from build123d import *

# Parameters (mm, degrees)
F0_R     = 68.9341581071
F1_DEPTH = 6.35
F2_R     = 25.775239711
F3_DEPTH = 3.81
F5_R     = 16.9134232358
F6_DEPTH = 3.81


# Not quite as in the source:
# - a feature names something its author has since deleted; it is built from what else it names


with BuildPart() as f1:
    # F0 (on Top) → F1 (new body)
    with BuildSketch(Plane.XY):
        Circle(F0_R)
    extrude(amount=F1_DEPTH)

    # F2 (on face) → F3 (cut)
    with BuildSketch(Plane.XY.offset(6.35)):
        Circle(F2_R)
    extrude(amount=-F3_DEPTH, mode=Mode.SUBTRACT)

    # F5 (on face) → F6 (cut)
    with BuildSketch(Plane.XY.offset(6.35)):
        with Locations((-42.6894489161, -25.2584252012)):
            Circle(F5_R)
        with Locations((-37.2139550745, 32.7947959304)):
            Circle(F5_R)
        with Locations((19.6899598242, 45.5267237403)):
            Circle(F5_R)
        with Locations((49.383019483, -4.6577332624)):
            Circle(F5_R)
        with Locations((10.8304246834, -48.405361207)):
            Circle(F5_R)
    extrude(amount=-F6_DEPTH, mode=Mode.SUBTRACT)


solid = f1.part
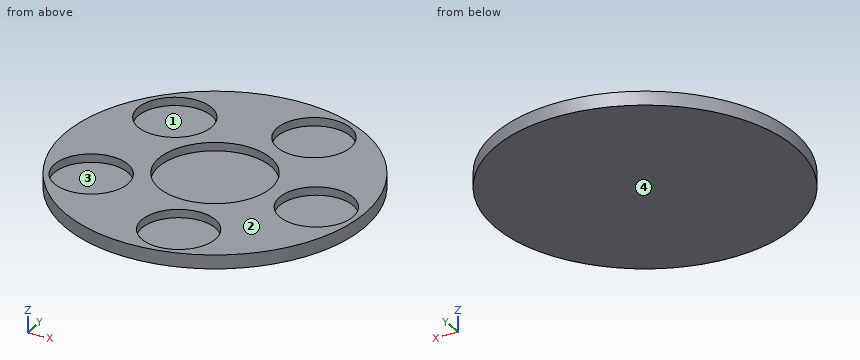
CAD build for the part. Positions are in the model's coordinates, mm. Face numbers are marked on the shaded views. A direction names the side the tool comes from. Give positions to 0.01 mm unless a question says otherwise; leave off trailing zeros. Order: outer loops, then holes, each group sorted by start corner. A loop starts at its lowest first (then second) coordinate and runs counter-clockwise, first axis right, second up. Notation, with made-up numbers: (-22.75, 77.5) - (5.25, 77.5) arc R10 cw to (5.25, 82.5) - close; hole circle Ø4 at (16.25, -36.5). An arc over 180 degrees is marked (long way). Answer in a Markdown table with one row per item.
1. Saw through at A-A, the plane z = 4.75. Give the cut face in (x, y), plus the area to 3 significant figures.
Data:
| item | result |
|---|---|
| outline | circle Ø137.87 at (0, 0); hole circle Ø33.83 at (-42.69, -25.26); hole circle Ø33.83 at (-37.21, 32.79); hole circle Ø51.55 at (0, 0); hole circle Ø33.83 at (10.83, -48.41); hole circle Ø33.83 at (19.69, 45.53); hole circle Ø33.83 at (49.38, -4.66) |
| area | 8,350 mm² |
2. Probe probe 1 along X at (y, z) = (9, 4.75); probe 2 along X at (y, z) = (31, 3.5); probe 3 along Y at (x, z) = (-52, 4). List the from-to ranges inside material, lowest first. Write a range as [from, to].
Data:
| item | result |
|---|---|
| probe 1 | x = [-68.34, -24.15], [24.15, 39.41], [59.36, 68.34] |
| probe 2 | x = [-61.57, -54.03], [-20.4, 11.03], [28.35, 61.57] |
| probe 3 | y = [-45.25, -39.38], [-11.14, 24.58], [41.01, 45.25] |
3. Saw through at B-B, the plane y = 7.5. Give the cut face in (x, z), plus the area to 3 significant figures.
Data:
| item | result |
|---|---|
| outline | (-68.52, 0) - (68.52, 0) - (68.52, 6.35) - (61.14, 6.35) - (61.14, 2.54) - (37.62, 2.54) - (37.62, 6.35) - (24.66, 6.35) - (24.66, 2.54) - (-24.66, 2.54) - (-24.66, 6.35) - (-68.52, 6.35) - close |
| area | 593 mm² |
4. Pull direction Y, two halves, no side cores. Call the marked faces 3 and 4: pulls with the +Y half, pulls with the -Y half, needs draft (parallel to the pull), parting line crosses it, or undercut.
Data:
| item | result |
|---|---|
| face 3 | undercut |
| face 4 | needs draft |
5. Saw through at D-D, the plane x = 23.5. Give the cut face in (y, z).
Data:
| item | result |
|---|---|
| outline | (-64.8, 0) - (64.8, 0) - (64.8, 6.35) - (62.01, 6.35) - (62.01, 2.54) - (29.05, 2.54) - (29.05, 6.35) - (10.59, 6.35) - (10.59, 2.54) - (-10.59, 2.54) - (-10.59, 6.35) - (-37.2, 6.35) - (-37.2, 2.54) - (-59.61, 2.54) - (-59.61, 6.35) - (-64.8, 6.35) - close |
6. Saw through at C-C, the plane x = 1. Give the cut face in (y, z).
Data:
| item | result |
|---|---|
| outline | (-68.93, 0) - (68.93, 0) - (68.93, 6.35) - (25.76, 6.35) - (25.76, 2.54) - (-25.76, 2.54) - (-25.76, 6.35) - (-34.64, 6.35) - (-34.64, 2.54) - (-62.17, 2.54) - (-62.17, 6.35) - (-68.93, 6.35) - close |
7. Flat gauge pins, fed straight in: pin 1 (1.5 mm diameter, centred on x = 37, z = 3.5, fed in from +Y); pin 2 (10 mm diameter, centred on x = -45, y = -18.5, fed in from +Z); pin 3 (3 mm diameter, centred on x = -20, z = 1, fed in from -Y). Where does each tip first touch, or does it go through?
Data:
| item | result |
|---|---|
| pin 1 | stops at y = 58.63 |
| pin 2 | stops at z = 2.54 |
| pin 3 | stops at y = -66.41 |
8. Tool access for the marked faces 1 and 2: list every direction of +Z, -Z, +X, -X, +Y, -Y with a clear straight run to the whole face (end or side of a thin tool).
Data:
| item | result |
|---|---|
| face 1 | +Z |
| face 2 | +Z, +X, -X, +Y, -Y |
